```python
from build123d import *

# Parameters (mm, degrees)
SKETCH1_W           = 50.8
SKETCH1_H           = 50.8
SKETCH1_R           = 1.905
SKETCH1_R_2         = 4.625
BOSS_EXTRUDE1_DEPTH = 6.35
FILLET1_R           = 2.54
SKETCH4_R           = 1.905
CUT_EXTRUDE3_DEPTH  = 3.175
BOSS_EXTRUDE2_DEPTH = 6.35
SKETCH6_R           = 25.4
SKETCH6_R_2         = 16.1
BOSS_EXTRUDE3_DEPTH = 7.366


with BuildPart() as part:
    # Sketch1 → Boss-Extrude1 (new body)
    with BuildSketch(Plane(origin=(0, 0, 0), x_dir=(1, 0, 0), z_dir=(0, 1, 0))):
        with Locations((25.4, 25.4)):
            Rectangle(SKETCH1_W, SKETCH1_H)
        with Locations(Location((4.490128061, 46.309871939, 0), (0, 0, 270))):
            Circle(SKETCH1_R, mode=Mode.SUBTRACT)
        with Locations(Location((4.490128061, 4.490128061, 0), (0, 0, 270))):
            Circle(SKETCH1_R, mode=Mode.SUBTRACT)
        with Locations(Location((46.309871939, 4.490128061, 0), (0, 0, 270))):
            Circle(SKETCH1_R, mode=Mode.SUBTRACT)
        with Locations(Location((46.309871939, 46.309871939, 0), (0, 0, 270))):
            Circle(SKETCH1_R, mode=Mode.SUBTRACT)
        with Locations(Location((25.4, 25.4, 0), (0, 0, 270))):
            Circle(SKETCH1_R_2, mode=Mode.SUBTRACT)
    extrude(amount=BOSS_EXTRUDE1_DEPTH)

    # Fillet1
    fillet1_edges = [part.edges().sort_by_distance(p)[0] for p in [
        (50.8, 3.175, -50.8),
        (50.8, 3.175, 0),
        (0, 3.175, 0),
        (0, 3.175, -50.8),
    ]]
    fillet(fillet1_edges, radius=FILLET1_R)

    # Sketch4 → Cut-Extrude3 (cut)
    with BuildSketch(Plane.XZ):
        with Locations(Location((4.490128061, -4.490128061, 0), (0, 0, 90))):
            Circle(SKETCH4_R)
        with BuildLine():
            Line((10.205128061, -4.490128061), (40.594871939, -4.490128061))
            ThreePointArc((40.594871939, -4.490128061), (42.268756685, -8.531243315), (46.309871939, -10.205128061))
            Line((46.309871939, -10.205128061), (46.309871939, -40.594871939))
            ThreePointArc((46.309871939, -40.594871939), (42.268756685, -42.268756685), (40.594871939, -46.309871939))
            Line((40.594871939, -46.309871939), (10.205128061, -46.309871939))
            ThreePointArc((10.205128061, -46.309871939), (8.531243315, -42.268756685), (4.490128061, -40.594871939))
            Line((4.490128061, -40.594871939), (4.490128061, -10.205128061))
            ThreePointArc((4.490128061, -10.205128061), (8.531243315, -8.531243315), (10.205128061, -4.490128061))
        make_face()
    extrude(amount=-CUT_EXTRUDE3_DEPTH, mode=Mode.SUBTRACT)

    # Sketch5 → Boss-Extrude2 (add)
    with BuildSketch(Plane(origin=(0, 6.35, 0), x_dir=(1, 0, 0), z_dir=(0, 1, 0))):
        with BuildLine():
            Line((63.5, 2.54), (63.5, 48.26))
            ThreePointArc((63.5, 48.26), (59.036307345, 59.036307345), (48.26, 63.5))
            Line((48.26, 63.5), (2.54, 63.5))
            ThreePointArc((2.54, 63.5), (-8.236307345, 59.036307345), (-12.7, 48.26))
            Line((-12.7, 48.26), (-12.7, 2.54))
            ThreePointArc((-12.7, 2.54), (-8.236307345, -8.236307345), (2.54, -12.7))
            Line((2.54, -12.7), (48.26, -12.7))
            ThreePointArc((48.26, -12.7), (59.036307345, -8.236307345), (63.5, 2.54))
        make_face()
        with BuildLine():
            Line((50.8, 2.54), (50.8, 48.26))
            ThreePointArc((50.8, 48.26), (50.056051224, 50.056051224), (48.26, 50.8))
            Line((48.26, 50.8), (2.54, 50.8))
            ThreePointArc((2.54, 50.8), (0.743948776, 50.056051224), (0, 48.26))
            Line((0, 48.26), (0, 2.54))
            ThreePointArc((0, 2.54), (0.743948776, 0.743948776), (2.54, 0))
            Line((2.54, 0), (48.26, 0))
            ThreePointArc((48.26, 0), (50.056051224, 0.743948776), (50.8, 2.54))
        make_face(mode=Mode.SUBTRACT)
    extrude(amount=-BOSS_EXTRUDE2_DEPTH)

    # Sketch6 → Boss-Extrude3 (add)
    with BuildSketch(Plane(origin=(0, 6.35, 0), x_dir=(1, 0, 0), z_dir=(0, 1, 0))):
        with Locations(Location((25.4, 25.4, 0), (0, 0, 270))):
            Circle(SKETCH6_R)
        with Locations(Location((25.4, 25.4, 0), (0, 0, 270))):
            Circle(SKETCH6_R_2, mode=Mode.SUBTRACT)
    extrude(amount=BOSS_EXTRUDE3_DEPTH)


solid = part.part
```
Geometry: final body of the model. Coordinates: model frame, mm. A direction names the side the tool comes from. Coordinates: 2 decimals unless noted, no trailing zeros. Order: outer loops, then holes, each group sorted by start corner. A loop starts at its lowest first (then second) coordinate and runs counter-clockwise, first axis right, second up. Notation, with made-up numbers: (-33, 33.5) - (16, 33.5) arc R16 ccw to (16, 39.5) - close; hole circle Ø4 at (-20, 10). An arc over 180 degrees is marked (long way). Return JSON: item names as keys, results as strings. Group by question number.
1. Pull-direction query (X, two-part tool) for faces 4 (the face through (59.15, 3.22, -58.92)), 5 (the face through (8, 2, -9)), 6 (the face through (42, 0, -43)); classes: pulls with the +X half, pulls with the -X half, needs draft (parallel to the pull), parting line crosses it, or undercut.
2. Cut plane B-B (z = -25.4). Output: boundary loops of the cut face in (x, y) (3 decimals), plus the area to 3 significant figures.
3. Set-up query: faces 1 (the face through (6.38, 3.13, -4.74)), 2 (the face through (29, 6.35, -22)), 3 (the face through (42.313, 1.565, -42.225)). Return all of +Z, -Z, +X, -X, +Y, -Y with unobstructed straight access to the full face (end or side cutting, diameter ignored); none if empty.
4. Pin query (flat end, axial travel): pin 1 (6 mm diameter, centred on x = 37.5, z = 2, fed in from -Y); pin 2 (10.5 mm diameter, centred on x = 25.4, z = -25.4, fed in from -Y) (3 decimals); pin 3 (4.5 mm diameter, centred on x = 4.49, z = -4.49, fed in from +Y); pin 4 (2 mm diameter, centred on y = 3.5, z = -52, fed in from -X). Return the tip coordinate at first contact, or that it passes through.
5. Cut plane C-C (x = 25.4). Output: boundary loops of the cut face in (y, z) (3 decimals), plus the area to 3 significant figures.
6. Cut plane D-D (y = 7.75). Output: boundary loops of the cut face in (x, z), plus the area to 3 significant figures.
7. Material intervals for line 1 along X through (y, z) = (4, -25.4) (3 decimals); line 2 along Z through (x, y) = (25.4, 4.45) (3 decimals); line 3 along Y through (x, z) = (39.5, -44.5) (3 decimals), sorted ascending. Write a range as [from, to].
8. Cut plane A-A (y = 1). Output: boundary loops of the cut face in (x, z) (3 decimals).
Resolved:
{
 "1": {"face 4": "pulls with the +X half", "face 5": "undercut", "face 6": "needs draft"},
 "2": {"outline": "(-12.7, 0) - (4.49, 0) - (4.49, 3.175) - (20.775, 3.175) - (20.775, 6.35) - (9.3, 6.35) - (9.3, 13.716) - (0, 13.716) - (0, 6.35) - (-12.7, 6.35) - close; (30.025, 3.175) - (46.31, 3.175) - (46.31, 0) - (63.5, 0) - (63.5, 6.35) - (50.8, 6.35) - (50.8, 13.716) - (41.5, 13.716) - (41.5, 6.35) - (30.025, 6.35) - close", "area": "459 mm²"},
 "3": {"face 1": "+Y, -Y", "face 2": "+Y", "face 3": "-Y"},
 "4": {"pin 1": "stops at y = 0", "pin 2": "stops at y = 3.175", "pin 3": "stops at y = 6.35", "pin 4": "stops at x = -12.45"},
 "5": {"outline": "(0, -63.5) - (6.35, -63.5) - (6.35, -50.8) - (13.716, -50.8) - (13.716, -41.5) - (6.35, -41.5) - (6.35, -30.025) - (3.175, -30.025) - (3.175, -46.31) - (0, -46.31) - close; (0, -4.49) - (3.175, -4.49) - (3.175, -20.775) - (6.35, -20.775) - (6.35, -9.3) - (13.716, -9.3) - (13.716, 0) - (6.35, 0) - (6.35, 12.7) - (0, 12.7) - close", "area": "459 mm²"},
 "6": {"outline": "circle Ø50.8 at (25.4, -25.4); hole circle Ø32.2 at (25.4, -25.4)", "area": "1,210 mm²"},
 "7": {"line 1": "x = [-12.7, 20.775], [30.025, 63.5]", "line 2": "z = [-63.5, -30.025], [-20.775, 12.7]", "line 3": "y = [3.175, 13.716]"},
 "8": {"outline": "(-12.7, -48.26) arc R15.24 ccw to (2.54, -63.5) - (48.26, -63.5) arc R15.24 ccw to (63.5, -48.26) - (63.5, -2.54) arc R15.24 ccw to (48.26, 12.7) - (2.54, 12.7) arc R15.24 ccw to (-12.7, -2.54) - close; hole circle Ø3.81 at (4.49, -46.31); hole circle Ø3.81 at (4.49, -4.49); hole (4.49, -40.595) arc R5.715 cw to (10.205, -46.31) - (40.595, -46.31) arc R5.715 cw to (46.31, -40.595) - (46.31, -10.205) arc R5.715 cw to (40.595, -4.49) - (10.205, -4.49) arc R5.715 cw to (4.49, -10.205) - close; hole circle Ø3.81 at (46.31, -46.31); hole circle Ø3.81 at (46.31, -4.49)"}
}
